For this review, take the finished solid that the model builds, in its own axes (mm). A direction names the side the tool comes from. Round coordinates to 2 decimals unless told otherwise and drop trailing zeros. Order: outer loops, then holes, each group sorted by start corner. A loop starts at its lowest first (then second) coordinate and runs counter-clockwise, first axis right, second up. Notation, with made-up numbers: M -2,-2 L 38,-2 A19 cw 38,28 Z; hole C 77.25,20.5 d5. An arc over 180 degrees is marked long. Answer as a JSON object with one key per item and string values.
from build123d import *

# Parameters (mm, degrees)
SKETCH1_R           = 0.9
SKETCH1_R_2         = 1.45
SKETCH1_R_3         = 7
SKETCH1_W           = 3.400011
SKETCH1_H           = 6.1
SKETCH1_W_2         = 3.4
BOSS_EXTRUDE2_DEPTH = 5.85
SKETCH2_R           = 1.25
CUT_EXTRUDE1_DEPTH  = 1


with BuildPart() as part:
    # Sketch1 → Boss-Extrude2 (new body)
    with BuildSketch(Plane.XY):
        with BuildLine():
            Line((669.21684417, 350.11545661), (648.4638119, 350.11545661))
            ThreePointArc((648.4638119, 350.11545661), (647.249496344, 349.612470637), (646.746510371, 348.398155081))
            Line((646.746510371, 348.398155081), (646.746510371, 313.132758138))
            ThreePointArc((646.746510371, 313.132758138), (647.249496344, 311.918442582), (648.4638119, 311.41545661))
            Line((648.4638119, 311.41545661), (669.21684417, 311.41545661))
            Line((669.21684417, 311.41545661), (684.726521371, 311.41545661))
            ThreePointArc((684.726521371, 311.41545661), (691.176521371, 317.86545661), (684.726521371, 324.31545661))
            Line((684.726521371, 324.31545661), (675.776521371, 324.31545661))
            ThreePointArc((675.776521371, 324.31545661), (669.326521371, 330.76545661), (675.776521371, 337.21545661))
            Line((675.776521371, 337.21545661), (684.726521371, 337.21545661))
            ThreePointArc((684.726521371, 337.21545661), (691.176521371, 343.66545661), (684.726521371, 350.11545661))
            Line((684.726521371, 350.11545661), (669.21684417, 350.11545661))
        make_face()
        with Locations((684.726521371, 343.66545661)):
            Circle(SKETCH1_R, mode=Mode.SUBTRACT)
        with Locations((684.726521371, 317.86545661)):
            Circle(SKETCH1_R, mode=Mode.SUBTRACT)
        with Locations((658.726521371, 317.46545661)):
            Circle(SKETCH1_R_2, mode=Mode.SUBTRACT)
        with Locations((658.726521371, 330.76545661)):
            Circle(SKETCH1_R_3, mode=Mode.SUBTRACT)
        with Locations((651.446515871, 344.06545661)):
            Rectangle(SKETCH1_W, SKETCH1_H, mode=Mode.SUBTRACT)
        with Locations((653.576521371, 317.46545661)):
            Rectangle(SKETCH1_W_2, SKETCH1_H, mode=Mode.SUBTRACT)
        with Locations((666.006526871, 344.06545661)):
            Rectangle(SKETCH1_W, SKETCH1_H, mode=Mode.SUBTRACT)
        with Locations((663.876521371, 317.46545661)):
            Rectangle(SKETCH1_W_2, SKETCH1_H, mode=Mode.SUBTRACT)
    extrude(amount=BOSS_EXTRUDE2_DEPTH)

    # Sketch2 → Cut-Extrude1 (cut)
    with BuildSketch(Plane.XY.offset(5.85)):
        with Locations((668.826521371, 317.46545661)):
            Circle(SKETCH2_R)
    extrude(amount=-CUT_EXTRUDE1_DEPTH, mode=Mode.SUBTRACT)


solid = part.part
1) Add section B-B on y = 345.5. State the section outline as (x, z) points.
Geometry check:
{"outline": "M 646.75,0 L 649.75,0 L 649.75,5.85 L 646.75,5.85 Z; M 653.15,0 L 664.31,0 L 664.31,5.85 L 653.15,5.85 Z; M 667.71,0 L 690.91,0 L 690.91,5.85 L 667.71,5.85 Z"}
2) Machinability: for faces 1 (the flat face through (666, 347.115, 3)), 2 (the cylindrical face through (670.02, 317.84, 5.36)), 3 (the flat face through (680, 324.315, 3)), which of the approach directions +Z, -Z, +X, -X, +Y, -Y give a long, thin tool a straight path to every point of the face, cutting with its end or side? Answer none if there is none.
Geometry check:
{"face 1": "+Z, -Z", "face 2": "+Z", "face 3": "+Z, -Z, +X"}
3) Insertion check: P1, Ø1, axis at x = 665, y = 339, coming from the -Z side. The pin has a flat end and moves straight along its axis. Give the tip position at first contact, or say it passes through.
Geometry check:
{"P1": "stops at z = 0"}
4) Add section A-A on x = 682.5. State the section outline as (y, z) points.
Geometry check:
{"outline": "M 311.42,0 L 324.32,0 L 324.32,5.85 L 311.42,5.85 Z; M 337.22,0 L 350.12,0 L 350.12,5.85 L 337.22,5.85 Z"}
5) Add section D-D on x = 659.5. State the section outline as (y, z) points, and give its area (3 significant figures).
Geometry check:
{"outline": "M 311.42,0 L 316.24,0 L 316.24,5.85 L 311.42,5.85 Z; M 318.69,0 L 323.81,0 L 323.81,5.85 L 318.69,5.85 Z; M 337.72,0 L 350.12,0 L 350.12,5.85 L 337.72,5.85 Z", "area": "131 mm²"}
6) For L1, parallel to Y at x = 685, z = 2.1; L2, parallel to Y at x = 667.5, z = 2.8; L3, parallel to X at y = 318, z = 3.3, list the stretches that pass through material, from the lowest coordinate up.
Geometry check:
{"L1": "y = 311.42 to 317.01, 318.72 to 324.31, 337.22 to 342.81, 344.52 to 350.11", "L2": "y = 311.42 to 341.02, 347.12 to 350.12", "L3": "x = 646.75 to 651.88, 655.28 to 657.38, 660.07 to 662.18, 665.58 to 683.84, 685.62 to 691.18"}
7) Mouldability with a two-part tool opening along X and no side actions: class faces 4 (the flat face through (653.147, 344, 3)), 5 (the flat face through (666, 311.415, 3)), 6 (the cylindrical face through (691.175, 317.724, 2.884)) as +X half, -X half, draft (parallel to the pull), parting line (faces both ways), or undercut.
Geometry check:
{"face 4": "undercut", "face 5": "draft", "face 6": "+X half"}
8) Add section C-C on y = 327.5. State the section outline as (x, z) points.
Geometry check:
{"outline": "M 646.75,0 L 652.53,0 L 652.53,5.85 L 646.75,5.85 Z; M 664.92,0 L 670.21,0 L 670.21,5.85 L 664.92,5.85 Z"}
